from build123d import *

# Parameters (mm, degrees)
SKETCH1_W           = 20
SKETCH1_H           = 100
BOSS_EXTRUDE1_DEPTH = 5
FILLET1_R           = 10
SKETCH2_R           = 4.95
BOSS_EXTRUDE2_DEPTH = 4.6
SKETCH2_4_R         = 5.05
CUT_EXTRUDE1_DEPTH  = 5
SKETCH4_W           = 10
SKETCH4_H           = 50
CUT_EXTRUDE2_DEPTH  = 5


with BuildPart() as part:
    # Sketch1 → Boss-Extrude1 (new body)
    with BuildSketch(Plane(origin=(0, 0, 0), x_dir=(1, 0, 0), z_dir=(0, 1, 0))):
        with Locations((-13.333333333, 18.974358974)):
            Rectangle(SKETCH1_W, SKETCH1_H)
    extrude(amount=BOSS_EXTRUDE1_DEPTH)

    # Fillet1
    fillet1_edges = [part.edges().sort_by_distance(p)[0] for p in [
        (-23.333333333, 2.5, -68.974358974),
        (-3.333333333, 2.5, -68.974358974),
        (-23.333333333, 2.5, 31.025641026),
        (-3.333333333, 2.5, 31.025641026),
    ]]
    fillet(fillet1_edges, radius=FILLET1_R - 0.0001)  # a hair under: the kernel refuses the full size

    # Sketch2 → Boss-Extrude2 (add)
    with BuildSketch(Plane(origin=(0, 5, 0), x_dir=(1, 0, 0), z_dir=(0, 1, 0))):
        with Locations(Location((-13.333333333, -21.025641026, 0), (0, 0, 90))):
            Circle(SKETCH2_R)
    extrude(amount=BOSS_EXTRUDE2_DEPTH)

    # Sketch2<4> → Cut-Extrude1 (cut)
    with BuildSketch(Plane(origin=(0, 5, 0), x_dir=(1, 0, 0), z_dir=(0, 1, 0))):
        with Locations(Location((-13.333333333, 58.974358974, 0), (0, 0, 270))):
            Circle(SKETCH2_4_R)
    extrude(amount=-CUT_EXTRUDE1_DEPTH, mode=Mode.SUBTRACT)

    # Sketch4 → Cut-Extrude2 (cut)
    with BuildSketch(Plane(origin=(0, 5, 0), x_dir=(1, 0, 0), z_dir=(0, 1, 0))):
        with Locations((-13.333333333, 18.974358974)):
            Rectangle(SKETCH4_W, SKETCH4_H)
    extrude(amount=-CUT_EXTRUDE2_DEPTH, mode=Mode.SUBTRACT)


solid = part.part
Geometry: final body of the model. Coordinates: model frame, mm. A direction names the side the tool comes from. Give positions to 0.01 mm unless a question says otherwise; leave off trailing zeros. Loops run counter-clockwise (first coordinate to the right, second up) from the corner with the lowest first, then second, coordinate; pieces in that order, holes last. Notation, with made-up numbers: M -36,38.25 L -25,38.25 A30 ccw -25,62.25 Z; hole C 50,-12.75 d6. An arc over 180 degrees is marked long. Put each result on its own line as item: value.
1) Mould query, pull axis X, two halves, no side actions, for faces 1 (the flat face through (-13, 3, -43.974)), 2 (the cylindrical face through (-14.8, 7.3, 16.3)), 3 (the cylindrical face through (-6.185, 2.535, -65.967)). Classes: released by +X, released by -X, zero draft, split by the parting line, or undercut.
Computed values:
face 1: undercut
face 2: split by the parting line
face 3: released by +X
2) Cut plane B-B, the plane x = -15.5. Return the cut outline in (y, z).
Computed values:
outline: M 0,-68.74 L 5,-68.74 L 5,-63.54 L 0,-63.54 Z; M 0,-54.41 L 5,-54.41 L 5,-43.97 L 0,-43.97 Z; M 0,6.03 L 5,6.03 L 5,16.58 L 9.6,16.58 L 9.6,25.48 L 5,25.48 L 5,30.79 L 0,30.79 Z
3) Cut plane A-A, the plane z = -19. Return the cut outline in (x, y), plus the area to 3 significant figures.
Computed values:
outline: M -23.33,0 L -18.33,0 L -18.33,5 L -23.33,5 Z; M -8.33,0 L -3.33,0 L -3.33,5 L -8.33,5 Z
area: 50.0 mm^2
4) Material intervals for L1, parallel to X at y = 2.5, z = -18.5; L2, parallel to Z at x = -10.75, y = 1; L3, parallel to Z at x = -16.75, y = 3, sorted ascending. Write a range as from..to.
Computed values:
L1: x = -23.33..-18.33, -8.33..-3.33
L2: z = -68.63..-63.31, -54.64..-43.97, 6.03..30.69
L3: z = -68.37..-62.69, -55.26..-43.97, 6.03..30.42
5) Reachability of faces 4 (the flat face through (-7, 0, -20)), 5 (the flat face through (-13, 3, 6.026)) from +Z, -Z, +X, -X, +Y, -Y: full face, straight path, thin tool, end or side. Return the list, or none.
Computed values:
face 4: +Z, -Z, +X, -X, -Y
face 5: +Y, -Y
6) First-contact query: P1, Ø1.5, axis at x = -17.5, z = -48.5, coming from the +Y side; P2, Ø11.5, axis at x = -13.33, z = -58.97, coming from the -Y side; P3, Ø2.5, axis at x = -11.5, y = 2, coming from the -Z side; P4, Ø1.5, axis at x = -11, y = 5.5, coming from the -Z side. Flat tips, straight axial feed; report the tip coordinate or a pass-through.
Computed values:
P1: stops at y = 5
P2: stops at y = 0
P3: stops at z = -68.96
P4: stops at z = -68.82
7) Cut plane C-C, the plane y = 1.75. Give the number of separate pieces and of enclosed holes in the cut face, plus the area to 3 significant figures.
Computed values:
separate pieces: 1
enclosed holes: 2
area: 1,330 mm^2
8) Cut plane D-D, the plane z = -62. Return the cut outline in (x, y), plus the area to 3 significant figures.
Computed values:
outline: M -22.86,0 L -17.38,0 L -17.38,5 L -22.86,5 Z; M -9.29,0 L -3.8,0 L -3.8,5 L -9.29,5 Z
area: 54.9 mm^2
